Read the model definition and answer for the solid it produces. Units are mm, in the model's axes. Coordinates: 2 decimals unless noted, no trailing zeros. Write each loop counter-clockwise with the first axis right and the second up, starting at its lowest first coordinate (ties: lowest second). Pieces come first, ordered by that corner, then holes.
Item 1: Straight lines are drawn through the part: probe 1 along Y at (x, z) = (14.35, 0); probe 2 along Z at (x, y) = (-12.5, 175.5); probe 3 along X at (y, z) = (1440.5, 10.5). For each, find the intervals that lie inside material, in ascending order.
Item 2: Section B-B (x = -6) is taken. Give the vertices of the cut face in (y, z).
Item 3: Section A-A (y = 627.5) is taken. Give the vertices of the cut face in (x, z).
Item 4: Each of these flat-tipped pins is pushed along its axis until it touches: P1, Ø12, axis at x = -6, z = 8.5, coming from the +Y side; P2, Ø12, axis at x = 6.5, z = -0.5, coming from the -Y side. Where does it stop, or does it pass through?
Autodesk Inventor part; units mm, degrees
ref_plane "YZ Plane" through (0, 0, 0) normal (1, 0, 0) x (0, 1, 0)
ref_plane "XZ Plane" through (0, 0, 0) normal (0, 1, 0) x (-1, 0, 0)
ref_plane "XY Plane" through (0, 0, 0) normal (0, 0, 1) x (1, 0, 0)
sketch "Sketch1" plane through (0, 0, 0) normal (0, 1, 0) x (-1, 0, 0)
  line L0 (-12, 14) -> (12, 14) construction
  line L1 (14, 12) -> (14, -12) construction
  line L2 (12, -14) -> (-12, -14) construction
  line L3 (-14, -12) -> (-14, 12) construction
  line L4 (-14, 14) -> (14, -14) construction
  line L5 (14, 14) -> (-14, -14) construction
  arc A0 (14, 12) -> (12, 14) centre (12, 12) ccw construction
  arc A1 (12, -14) -> (14, -12) centre (12, -12) ccw construction
  arc A2 (-14, -12) -> (-12, -14) centre (-12, -12) ccw construction
  arc A3 (-12, 14) -> (-14, 12) centre (-12, 12) ccw construction
  line L6 (-12, -15) -> (12, -15)
  arc A4 (12, -15) -> (15, -12) centre (12, -12) ccw
  line L7 (15, -12) -> (15, 12)
  arc A5 (15, 12) -> (12, 15) centre (12, 12) ccw
  line L8 (12, 15) -> (-12, 15)
  arc A6 (-12, 15) -> (-15, 12) centre (-12, 12) ccw
  line L9 (-15, 12) -> (-15, -12)
  arc A7 (-15, -12) -> (-12, -15) centre (-12, -12) ccw
  line L10 (13, -12) -> (13, 12)
  arc A8 (13, 12) -> (12, 13) centre (12, 12) ccw
  line L11 (12, 13) -> (-12, 13)
  arc A9 (-12, 13) -> (-13, 12) centre (-12, 12) ccw
  line L12 (-13, 12) -> (-13, -12)
  arc A10 (-13, -12) -> (-12, -13) centre (-12, -12) ccw
  line L13 (-12, -13) -> (12, -13)
  arc A11 (12, -13) -> (13, -12) centre (12, -12) ccw
  point P0 (0, 0)
  point P1 (0, 0)
  point P2 (0, 0)
  dimension "d10" = 2
  dimension "depth" = 30
  dimension "width" = 30
  dimension "thickness" = 2
extrude "Extrusion1" add sketch "Sketch1" along normal blind 2000
ref_plane "Work Plane1" through (0, 1000, 0) normal (0, -1, 0) x (1, 0, 0)
sketch "Sketch3" plane through (12, 0, -15) normal (0, 0, -1) x (-1, 0, 0)
  line L0 (12, -400) -> (12, 2400) construction
  circle A0 centre (-3, 1000) radius 985
  point P0 (12, 0)
  dimension "d29" = 1970
  dimension "d31" = 1000
  dimension "d34" = 15
extrude "Extrusion2" cut sketch "Sketch3" against normal through all keep common part
sketch "Sketch4" plane through (15, 15, 12) normal (1, 0, 0) x (0, 0, -1)
  line L0 (33.0025, 985) -> (-9.0025, 985) construction
  line L1 (12, -412.0004) -> (12, 2367.0022)
  point P0 (12, -15)
  point P1 (12, 235)
  point P2 (12, 985)
  point P3 (12, 1735)
  point P4 (12, 735)
  point P5 (12, 1235)
  dimension "d35" = 1500
  dimension "d36" = 500
hole "Hole2" at (15, 250, 0) at (15, 1750, 0) at (15, 750, 0) at (15, 1250, 0) direction (-1, 0, 0) diameter 8 depth 40 tip angle 118
equation "\"d10\" = thickness"
properties part number "podest duzy profil 1" material "Steel"
Established:
1. probe 1: y = 15 to 246, 254 to 746, 754 to 1246, 1254 to 1746, 1754 to 1985
1. probe 2: z = -14.96 to -12.87, 12.87 to 14.96
1. probe 3: x = -15 to -13, 13 to 15
2. outline: (15.22, -15) - (1984.78, -15) - (1984.78, -13) - (15.22, -13) - close; (15.22, 13) - (1984.78, 13) - (1984.78, 15) - (15.22, 15) - close
3. outline: (-15, -12) arc R3 ccw to (-12, -15) - (12, -15) arc R3 ccw to (15, -12) - (15, 12) arc R3 ccw to (12, 15) - (-12, 15) arc R3 ccw to (-15, 12) - close; hole (-13, -12) arc R1 ccw to (-12, -13) - (12, -13) arc R1 ccw to (13, -12) - (13, 12) arc R1 ccw to (12, 13) - (-12, 13) arc R1 ccw to (-13, 12) - close
4. P1: stops at y = 1984.85
4. P2: passes through
